Build history of the part. All positions in model axes, mm. A direction names the side the tool comes from. Round coordinates to 2 decimals unless told otherwise and drop trailing zeros. Write each loop counter-clockwise with the first axis right and the second up, starting at its lowest first coordinate (ties: lowest second). Pieces come first, ordered by that corner, then holes. Notation, with made-up numbers: (55, -26) - (93, -26) arc R27 cw to (93, -9) - close; hole circle Ø8 at (-17, 56.5). An arc over 180 degrees is marked (long way). One line per question, with ' | ' between items.
from build123d import *

# Parameters (mm, degrees)
SKETCH1_W                  = 15.875
SKETCH1_H                  = 15.875
BOSS_EXTRUDE1_DEPTH        = 57.15
CUT_EXTRUDE1_DEPTH         = 60.842643919
CUT_EXTRUDE1_DEPTH_BACK    = 60.842643919
F_12_CLEARANCE_HOLE1_D     = 5.7912
F_12_CLEARANCE_HOLE1_DEPTH = 42.07002
F_12_CLEARANCE_HOLE1_TIP   = 1.739852008
F_12_24_TAPPED_HOLE1_D     = 4.4958


with BuildPart() as part:
    # Sketch1 → Boss-Extrude1 (new, symmetric)
    with BuildSketch(Plane.XY):
        Rectangle(SKETCH1_W, SKETCH1_H)
    extrude(amount=BOSS_EXTRUDE1_DEPTH, both=True)

    # Sketch2 → Cut-Extrude1 (cut, two sides: drawn at the far end of the back side and taken through both)
    with BuildSketch(Plane(origin=(0, 7.9375, 0), x_dir=(1, 0, 0), z_dir=(0, 1, 0)).offset(-CUT_EXTRUDE1_DEPTH_BACK)):
        Polygon((66.547875099, 129.510772403), (7.9375, 4.7625), (5.699938661, 0), (7.9375, -4.7625), (66.547875099, -129.510772403), (342.209316267, -129.510772403), (342.209316267, 129.510772403), align=None)
    extrude(amount=CUT_EXTRUDE1_DEPTH + CUT_EXTRUDE1_DEPTH_BACK, mode=Mode.SUBTRACT)

    # #12 Clearance Hole1
    with Locations(Plane(origin=(7.9375, 0, 0), x_dir=(0, 0, -1), z_dir=(1, 0, 0))):
        with Locations((28.575, 0), (-28.575, 0)):
            Hole(F_12_CLEARANCE_HOLE1_D / 2, depth=F_12_CLEARANCE_HOLE1_DEPTH)
            with Locations((0, 0, -(F_12_CLEARANCE_HOLE1_DEPTH + F_12_CLEARANCE_HOLE1_TIP / 2))):  # 118° drill point
                Cone(0, F_12_CLEARANCE_HOLE1_D / 2, F_12_CLEARANCE_HOLE1_TIP, mode=Mode.SUBTRACT)

    # #12-24 Tapped Hole1 (through all)
    with Locations(Plane(origin=(0, -7.9375, 0), x_dir=(-1, 0, 0), z_dir=(0, -1, 0))):
        with Locations((0, 49.653581933)):
            Hole(F_12_24_TAPPED_HOLE1_D / 2)


solid = part.part
Q1. Drill centre lines: L1, parallel to Z at x = -4.75, y = -0.5; L2, parallel to Z at x = 0, y = -1; L3, parallel to Z at x = 4, y = 1.5. Where is each one in solid material? Low to high. Write a range as from..to.
Found:
L1: -57.15..-31.43, -25.72..25.72, 31.43..57.15 | L2: -57.15..-51.9, -47.41..-31.29, -25.86..25.86, 31.29..57.15 | L3: -57.15..-31.05, -26.1..26.1, 31.05..57.15
Q2. Which spindle directions (+Z, -Z, +X, -X, +Y, -Y) get a long thin tool onto all of the face, cutting with end or side? Do faces 5 (the flat face through (0, -7.938, 1)), 6 (the flat face through (6.834, -0.111, -2.415)). Say none if no direction does.
Found:
face 5: +Z, -Z, +X, -X, -Y | face 6: +X, +Y, -Y
Q3. Saw through at D-D, the plane z = 2.5. List the corners of the cut face in (x, y), then the cut area to 3 significant figures.
Found:
outline: (-7.94, -7.94) - (6.87, -7.94) - (6.87, 7.94) - (-7.94, 7.94) - close | area: 235 mm^2
Q4. Pull direction Z, two halves, no side cores. Call faces 1 (the flat face through (0, 0, -57.15)), 2 (the flat face through (6.803, -0.111, 2.348)), 3 (the flat face through (7.938, 2, 31)), 4 (the cylindrical face through (-0.111, 0.127, 25.682)): +Z half, -Z half, draft (parallel to the pull), parting line (faces both ways), or undercut.
Found:
face 1: -Z half | face 2: undercut | face 3: draft | face 4: undercut
Q5. Saw through at B-B, the plane y = 1. List the corners of the cut face in (x, z).
Found:
outline: (-7.94, -57.15) - (7.94, -57.15) - (7.94, -31.29) - (-7.94, -31.29) - close; (-7.94, -25.86) - (7.94, -25.86) - (7.94, -4.76) - (5.7, 0) - (7.94, 4.76) - (7.94, 25.86) - (-7.94, 25.86) - close; (-7.94, 31.29) - (7.94, 31.29) - (7.94, 57.15) - (-7.94, 57.15) - close; hole circle Ø4.5 at (0, -49.65)
Q6. Saw through at A-A, the plane x = 0. State how many separate pieces and enclosed holes the cut face has, then the cut area to 3 significant figures.
Found:
separate pieces: 2 | enclosed holes: 2 | area: 1,690 mm^2
